Design review of the part built by this model. Coordinates are the model's own, in mm. A direction names the side the tool comes from. Round coordinates to 2 decimals unless told otherwise and drop trailing zeros. Write each loop counter-clockwise with the first axis right and the second up, starting at its lowest first coordinate (ties: lowest second). Pieces come first, ordered by that corner, then holes. Notation, with made-up numbers: M 13.5,-12.75 L 62.5,-12.75 A15 ccw 62.5,9.25 Z; hole C 58,40 d6. An arc over 180 degrees is marked long. One line per question, with ' | ' between items. Start each with the question number.
Item 1: Draft analysis for pull direction X (two halves, no side actions). For faces 6 (the face through (4, -38, 1)), 7 (the face through (7, -32, 1)), 8 (the face through (-10, -35, 2)), state which applies: released by +X, released by -X, zero draft, split by the parting line, or undercut.
Item 2: Machinability: for faces 1 (the face through (-9, -33.544, 2)), 2 (the face through (-3, -36.544, 2)), 3 (the face through (4.5, 5, 1)), 4 (the face through (7, -38, 1)), 5 (the face through (-7, -38, 1)), which of the approach directions +Z, -Z, +X, -X, +Y, -Y give a long, thin tool a straight path to every point of the face, cutting with its end or side? Answer none if there is none.
Item 3: Add section D-D, the plane y = 30. State the section outline as (x, z) points, and give its area (3 significant figures).
Item 4: Add section C-C, the plane x = 6. State the section outline as (y, z) points.
Item 5: Add section B-B, the plane z = 0.6. State the section outline as (x, y) points.
Item 6: Insertion check: pin 1 Ø1.5 at (x, z) = (0, 1.5) entering from -Y; pin 2 Ø1.5 at (y, z) = (-37.5, 2) entering from +X; pin 3 Ø1.5 at (y, z) = (8, 1.5) entering from -X. Each pin has a flat end and moves straight along its axis. Give the tip position at first contact, or say it passes through.
Item 7: For L1, parallel to X at y = -35.5, z = 2.8; L2, parallel to X at y = -21, z = 0.65; L3, parallel to Y at x = 9.25, z = 0.2, list the stretches that pass through material, from the lowest coordinate up.
Item 8: Add section A-A, the plane y = 2. State the section outline as (x, z) points.
```python
from build123d import *

# Parameters (mm, degrees)
EXTRUDE_1_DEPTH     = 3
SKETCH_2_W          = 3
SKETCH_2_H          = 36.493999941
CUT_EXTRUDE_1_DEPTH = 3
SKETCH_3_W          = 3
SKETCH_3_H          = 3
EXTRUDE_2_DEPTH     = 3
SKETCH_5_W          = 2.5
SKETCH_5_H          = 3.1
EXTRUDE_3_DEPTH     = 3


with BuildPart() as part:
    # 스케치1 → 보스-돌출1 (new body)
    with BuildSketch(Plane.XY):
        Polygon((-4.5, 39.543999941), (4.5, 39.543999941), (4.5, -30.443999941), (7, -30.443999941), (7, -39.543999941), (4, -39.543999941), (4, -33.443999941), (-4, -33.443999941), (-4, -39.543999941), (-7, -39.543999941), (-7, -30.443999941), (-4.5, -30.443999941), align=None)
    extrude(amount=EXTRUDE_1_DEPTH)

    # 스케치2 → 컷-돌출1 (cut)
    with BuildSketch(Plane(origin=(0, 0, 0), x_dir=(-1, 0, 0), z_dir=(0, 0, -1))):
        with Locations((0, -15.196999971)):
            Rectangle(SKETCH_2_W, SKETCH_2_H)
    extrude(amount=-CUT_EXTRUDE_1_DEPTH, mode=Mode.SUBTRACT)

    # 스케치3 → 보스-돌출2 (add)
    with BuildSketch(Plane.XY.offset(3)):
        with Locations((-8.5, -35.043999941)):
            Rectangle(SKETCH_3_W, SKETCH_3_H)
        with Locations((8.5, -35.043999941)):
            Rectangle(SKETCH_3_W, SKETCH_3_H)
    extrude(amount=-EXTRUDE_2_DEPTH)

    # 스케치5 → 보스-돌출3 (add)
    with BuildSketch(Plane.XY.offset(3)):
        with Locations((-2.75, -34.993999941)):
            Rectangle(SKETCH_5_W, SKETCH_5_H)
        with Locations((2.75, -34.993999941)):
            Rectangle(SKETCH_5_W, SKETCH_5_H)
    extrude(amount=-EXTRUDE_3_DEPTH)


solid = part.part
```
Computed values:
1) face 6: undercut | face 7: released by +X | face 8: released by -X
2) face 1: +Z, -Z, -X, +Y | face 2: +Z, -Z, -Y | face 3: +Z, -Z, +X, +Y | face 4: +Z, -Z, +X, -Y | face 5: +Z, -Z, -X, -Y
3) outline: M -4.5,0 L 4.5,0 L 4.5,3 L -4.5,3 Z | area: 27.0 mm^2
4) outline: M -39.54,0 L -30.44,0 L -30.44,3 L -39.54,3 Z
5) outline: M -10,-36.54 L -7,-36.54 L -7,-39.54 L -4,-39.54 L -4,-36.54 L -1.5,-36.54 L -1.5,3.05 L 1.5,3.05 L 1.5,-36.54 L 4,-36.54 L 4,-39.54 L 7,-39.54 L 7,-36.54 L 10,-36.54 L 10,-33.54 L 7,-33.54 L 7,-30.44 L 4.5,-30.44 L 4.5,39.54 L -4.5,39.54 L -4.5,-30.44 L -7,-30.44 L -7,-33.54 L -10,-33.54 Z
6) pin 1: stops at y = 3.05 | pin 2: stops at x = 7 | pin 3: stops at x = -4.5
7) L1: x = -10 to -1.5, 1.5 to 10 | L2: x = -4.5 to -1.5, 1.5 to 4.5 | L3: y = -36.54 to -33.54
8) outline: M -4.5,0 L -1.5,0 L -1.5,3 L -4.5,3 Z; M 1.5,0 L 4.5,0 L 4.5,3 L 1.5,3 Z
